```python
from build123d import *

# Parameters (mm, degrees)
SKETCH1_W           = 100
SKETCH1_H           = 100
SKETCH1_R           = 10
SKETCH1_RX          = 11.867112324
SKETCH1_RY          = 5.7171528
SKETCH1_W_2         = 20
SKETCH1_H_2         = 20
BOSS_EXTRUDE1_DEPTH = 10


with BuildPart() as part:
    # Sketch1 → Boss-Extrude1 (new body)
    with BuildSketch(Plane(origin=(0, 0, 0), x_dir=(1, 0, 0), z_dir=(0, 1, 0))):
        Rectangle(SKETCH1_W, SKETCH1_H)
        Circle(SKETCH1_R, mode=Mode.SUBTRACT)
        with Locations(Location((-29.06507818, -29.06507818), (0, 0, 45))):
            Ellipse(SKETCH1_RX, SKETCH1_RY, mode=Mode.SUBTRACT)
        Polygon((-18.581564885, 30), (-24.355067577, 40), (-35.902072961, 40), (-41.675575653, 30), (-35.902072961, 20), (-24.355067577, 20), align=None, mode=Mode.SUBTRACT)
        with Locations((32.305830442, 32.305830442)):
            Rectangle(SKETCH1_W_2, SKETCH1_H_2, mode=Mode.SUBTRACT)
    extrude(amount=BOSS_EXTRUDE1_DEPTH)


solid = part.part
```
Source: CAD feature listing. Evaluate the final solid. Frame: model axes, mm. A direction names the side the tool comes from. Round coordinates to 2 decimals unless told otherwise and drop trailing zeros. Loops run counter-clockwise (first coordinate to the right, second up) from the corner with the lowest first, then second, coordinate; pieces in that order, holes last.
1. Contact query for a flat-ended pin moving along its axis: pin 1 (12 mm diameter, centred on x = 0, z = 0, fed in from -Y). Output: stop coordinate, or through.
2. Mould query, pull axis Z, two halves, no side actions, for faces 1 (the flat face through (-1, 5, -50)), 2 (the flat face through (-0.7, 0, 10.4)), 3 (the flat face through (-1, 5, 50)), 4 (the flat face through (42.306, 5, -32)). Classes: released by +Z, released by -Z, zero draft, split by the parting line, or undercut.
3. Section query A-A on x = 0. Output: boundary loops of the cut face in (y, z).
4. Access query for faces 5 (the flat face through (-38.83, 4.93, -25.07)), 6 (the flat face through (-0.7, 10, 10.4)). Directions: +Z, -Z, +X, -X, +Y, -Y. A direction counts if a zero-diameter tool reaches every point of the face in a straight line with its end or side. Return the directions, or none.
5. Section query B-B on z = -34. Output: boundary loops of the cut face in (x, y), and give its area (3 significant figures).
6. Section query D-D on x = -28. Give the number of separate pieces and of enclosed holes in the cut face, and give its area (3 significant figures).
7. Ray query, L1, parallel to Z at x = -35, y = 3.25; L2, parallel to X at y = 5.25, z = -39.5; L3, parallel to Z at x = 36.5, y = 7. Return the intervals inside material, ascending.
8. Section query C-C on z = 0. Output: boundary loops of the cut face in (x, y).
Answers below:
1. pin 1: passes through
2. face 1: released by -Z
2. face 2: zero draft
2. face 3: released by +Z
2. face 4: undercut
3. outline: (0, -50) - (10, -50) - (10, -10) - (0, -10) - close; (0, 10) - (10, 10) - (10, 50) - (0, 50) - close
4. face 5: +Y, -Y
4. face 6: +Z, -Z, +X, -X, +Y
5. outline: (-50, 0) - (-39.37, 0) - (-39.37, 10) - (-50, 10) - close; (-20.89, 0) - (22.31, 0) - (22.31, 10) - (-20.89, 10) - close; (42.31, 0) - (50, 0) - (50, 10) - (42.31, 10) - close
5. area: 615 mm2
6. separate pieces: 3
6. enclosed holes: 0
6. area: 655 mm2
7. L1: z = -50 to -40, -20 to 27.15, 38.38 to 50
7. L2: x = -50 to -36.19, -24.07 to 22.31, 42.31 to 50
7. L3: z = -50 to -42.31, -22.31 to 50
8. outline: (-50, 0) - (-10, 0) - (-10, 10) - (-50, 10) - close; (10, 0) - (50, 0) - (50, 10) - (10, 10) - close
